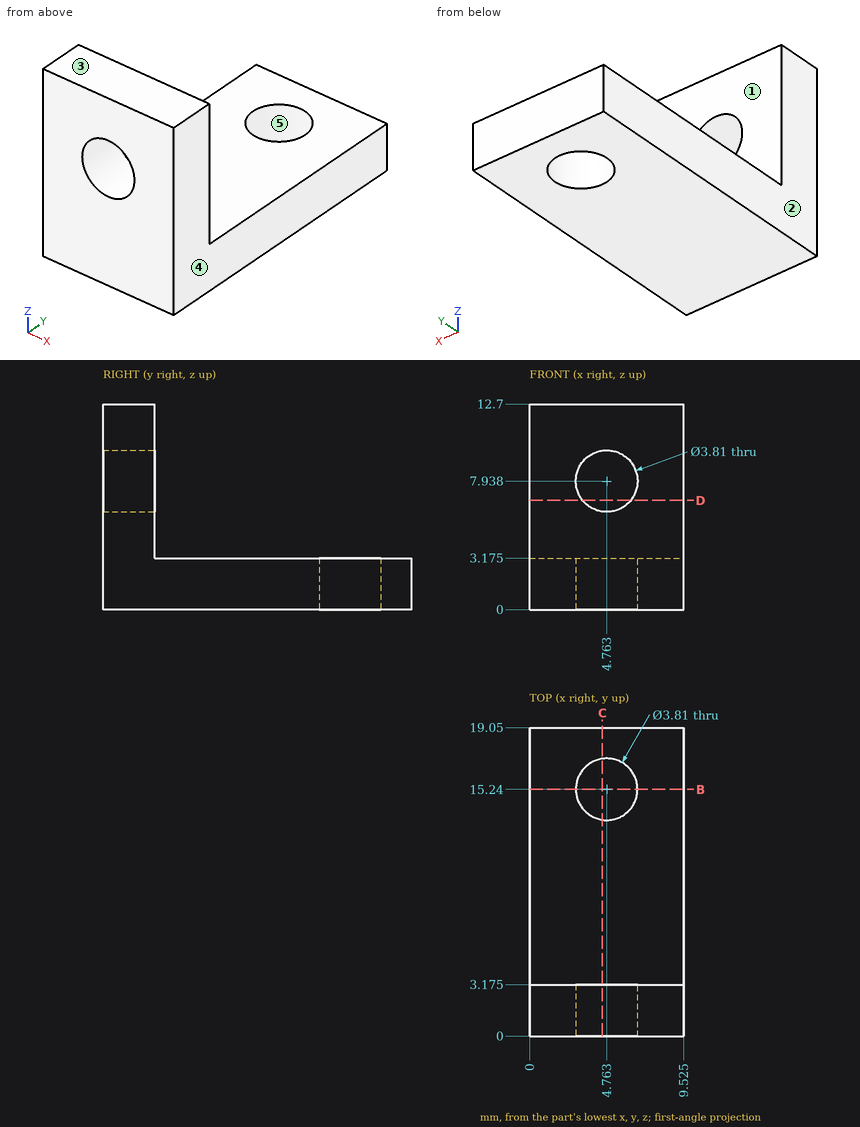
Study the drawing (mm; zero at the part's minimum x, y, z) and answer. A direction names the side the tool comes from. Give positions to 0.01 mm unless a question says otherwise; leave off trailing zeros. Order: outer loops, then holes, each group sorted by start corner. A loop starts at its lowest first (then second) coordinate and runs counter-clockwise, first axis right, second up. Notation, with made-up numbers: (65.5, 3.25) -> (108.5, 3.25) arc R17 ccw to (108.5, 31.25) -> close; hole circle Ø11 at (63, 48.25). An arc over 180 degrees is marked (long way). Write item = value, one per line.
1. A cutting plane is placed at C-C, the plane x = 4.5. Count the separate pieces of the cut face and the enclosed holes in it.
Numbers:
separate_pieces = 3
enclosed_holes = 0
2. Given pin 1 (1.5 mm diameter, centred on x = 5, z = 9.5, fed in from +Y) (1 decimal); pin 2 (4.5 mm diameter, centred on x = 4.76, y = 15.24, fed in from +Z) (1 decimal), each flat-ended and moving along its own axis, determine where each tip first touches the part or whether it passes through.
Numbers:
pin_1 = 3.2
pin_2 = 3.2
3. A cutting plane is placed at D-D, the plane z = 6.75. Write down the section's boundary in (x, y) (1 decimal).
Numbers:
outline = (0, 0) -> (3.3, 0) -> (3.3, 3.2) -> (0, 3.2) -> close; (6.3, 0) -> (9.5, 0) -> (9.5, 3.2) -> (6.3, 3.2) -> close
4. A cutting plane is placed at B-B, the plane y = 15.24. Write down the section's boundary in (x, z) (1 decimal).
Numbers:
outline = (0, 0) -> (2.9, 0) -> (2.9, 3.2) -> (0, 3.2) -> close; (6.7, 0) -> (9.5, 0) -> (9.5, 3.2) -> (6.7, 3.2) -> close
5. The mould has two halves that part along X. Classify the marked faces 3, 4 and 5: +X half, -X half, draft (parallel to the pull), parting line (faces both ways), or undercut.
Numbers:
face_3 = draft
face_4 = +X half
face_5 = undercut
6. For the marked faces 1 and 2, determine the directions among +Z, -Z, +X, -X, +Y, -Y from which every point of the face is accessible in a straight line to the end or side of a thin tool.
Numbers:
face_1 = +Z, +X, -X, +Y
face_2 = +Z, -Z, -X, +Y, -Y
7. Straight lines are drawn through the part: line 1 along X through (y, z) = (1, 8) (1 decimal); line 2 along Z through (x, y) = (3, 13) (1 decimal). For each, find the intervals that lie inside material, in ascending order.
Numbers:
line_1 = 0 to 2.9, 6.7 to 9.5
line_2 = 0 to 3.2
